The model under review builds one solid part; all positions refer to its coordinate system, in mm. Give positions to 0.01 mm unless a question says otherwise; leave off trailing zeros. Order: outer loops, then holes, each group sorted by start corner. A loop starts at its lowest first (then second) coordinate and runs counter-clockwise, first axis right, second up. Notation, with made-up numbers: (53, 71.25) - (100, 71.25) arc R4 cw to (100, 77.25) - close; hole circle Ø5 at (13, 61.25). An arc over 180 degrees is marked (long way). Use CSV: the item, a comma, the result in double quotes.
```python
from build123d import *

# Parameters (mm, degrees)
SKETCH1_R           = 12.7
BOSS_EXTRUDE1_DEPTH = 6.35
CUT_EXTRUDE1_REACH  = 21.05
SKETCH2_R           = 9.525
FILLET1_R           = 0.762


with BuildPart() as part:
    # Sketch1 → Boss-Extrude1 (new body)
    with BuildSketch(Plane(origin=(0, 0, 0), x_dir=(0, 0, -1), z_dir=(1, 0, 0))):
        Circle(SKETCH1_R)
    extrude(amount=BOSS_EXTRUDE1_DEPTH)

    # Sketch2 → Cut-Extrude1 (cut, up to next)
    with BuildSketch(Plane(origin=(6.35, 0, 0), x_dir=(0, 0, -1), z_dir=(1, 0, 0)), mode=Mode.PRIVATE) as cut_extrude1_sk1:
        Circle(SKETCH2_R)
    cut_extrude1_tool1 = extrude(cut_extrude1_sk1.sketch, amount=-CUT_EXTRUDE1_REACH, mode=Mode.PRIVATE) & part.part
    add(cut_extrude1_tool1.solids().sort_by_distance((6.35, 0, 0))[0], mode=Mode.SUBTRACT)

    # Fillet1
    fillet1_edges = [part.edges().sort_by_distance(p)[0] for p in [
        (6.35, 0, 9.525),
    ]]
    fillet(fillet1_edges, radius=FILLET1_R)


solid = part.part
```
Item 1: Wall thickness on L1, parallel to Y at x = 3.2, z = 0 (3 decimals); L2, parallel to Y at x = 3.5, z = -6; L3, parallel to Z at x = 6, y = 2.75: over which ranges is each line inside the solid? List them lowest first.
Results list:
L1,"y = -12.7 to -9.525, 9.525 to 12.7"
L2,"y = -11.19 to -7.4, 7.4 to 11.19"
L3,"z = -12.4 to -9.25, 9.25 to 12.4"
Item 2: Take a section at A-A, the plane y = 0. Give the boundary of the cut face in (x, z) (3 decimals), and give its area (3 significant figures).
Results list:
outline,"(0, -12.7) - (6.35, -12.7) - (6.35, -10.287) arc R0.762 ccw to (5.588, -9.525) - (0, -9.525) - close; (0, 9.525) - (5.588, 9.525) arc R0.762 ccw to (6.35, 10.287) - (6.35, 12.7) - (0, 12.7) - close"
area,"40.1 mm2"
Item 3: Mouldability with a two-part tool opening along Z and no side actions: class faces 1 (the face through (3.13, -12.4, 2.75)), 2 (the face through (0, 9, -5)), 3 (the face through (2.833, -5.796, 7.559)) as pulls with the +Z half, pulls with the -Z half, needs draft (parallel to the pull), parting line crosses it, or undercut.
Results list:
face 1,"parting line crosses it"
face 2,"needs draft"
face 3,"undercut"
Item 4: Take a section at D-D, the plane y = 11. Give the boundary of the cut face in (x, z).
Results list:
outline,"(0, -6.35) - (6.35, -6.35) - (6.35, 6.35) - (0, 6.35) - close"
Item 5: Take a section at C-C, the plane x = 2.5. Give the boundary of the cut face in (y, z) (3 decimals).
Results list:
outline,"circle Ø25.4 at (0, 0); hole circle Ø19.05 at (0, 0)"
Item 6: Clearance check with flat-ended pins moving along their axes: pin 1 (4 mm diameter, centred on y = 7, z = 1.5, fed in from -X); pin 2 (1.5 mm diameter, centred on x = 5.5, z = 3.5, fed in from +Y). State where each tip first meets the part, or that it passes through.
Results list:
pin 1,"passes through"
pin 2,"stops at y = 12.4"
